from build123d import *

# Parameters (mm, degrees)
BOSS_EXTRUDE1_DEPTH  = 9.525
M8_CLEARANCE_HOLE1_D = 9
FILLET1_R            = 10
CHAMFER1_SIZE        = 1


with BuildPart() as part:
    # Sketch1 → Boss-Extrude1 (new body)
    with BuildSketch(Plane(origin=(0, 0, 0), x_dir=(1, 0, 0), z_dir=(0, 1, 0))):
        Polygon((-20, 90), (-20, -20), (60, -20), (60, 10), (20, 10), (20, 90), align=None)
    extrude(amount=BOSS_EXTRUDE1_DEPTH)

    # M8 Clearance Hole1 (through all)
    with Locations(Plane(origin=(0, 9.525, 0), x_dir=(1, 0, 0), z_dir=(0, 1, 0))):
        with Locations((0, 0), (40, 0)):
            Hole(M8_CLEARANCE_HOLE1_D / 2)

    # Fillet1
    fillet1_edges = [part.edges().sort_by_distance(p)[0] for p in [
        (20, 4.7625, -10),
    ]]
    fillet(fillet1_edges, radius=FILLET1_R)

    # Chamfer1
    chamfer1_edges = [part.edges().sort_by_distance(p)[0] for p in [
        (20, 4.7625, -90),
        (60, 4.7625, -10),
        (60, 4.7625, 20),
        (-20, 4.7625, 20),
        (-20, 4.7625, -90),
    ]]
    chamfer(chamfer1_edges, length=CHAMFER1_SIZE)


solid = part.part
Check sheet for the modelled part. Datum: model origin and axes. Units: mm. A direction names the side the tool comes from. Coordinates: 2 decimals unless noted, no trailing zeros. Loops run counter-clockwise (first coordinate to the right, second up) from the corner with the lowest first, then second, coordinate; pieces in that order, holes last. Notation, with made-up numbers: (3, 13) -> (10, 13) arc R33 cw to (10, 41) -> close; hole circle Ø1 at (22, 26.5). An arc over 180 degrees is marked (long way). Write item = value, one per line. Start each with the question number.
1. Section check D-D on x = 0. Record the cut outline in (y, z) (3 decimals), then the cut area to 3 significant figures.
2. Material ranges on line 1 (X direction, y = 4.5, z = 1.5); line 2 (X direction, y = 3.25, z = 2); line 3 (Z direction, x = 0, y = 5), recorded low to high.
3. Section check C-C on y = 5.25. Record the cut outline in (x, z).
4. Depth check by flat-ended pin: P1, Ø1.5, axis at y = 6, z = -67, coming from the +X side; P2, Ø1, axis at x = 46.5, y = 6.5, coming from the -Z side; P3, Ø5, axis at x = 28.5, y = 7.5, coming from the -Z side. Enter the tip coordinate at first touch or a pass-through.
5. Tool access check on faces 4 (the flat face through (20, 5, -54)), 5 (the flat face through (0, 5, -90)). Record the directions out of +Z, -Z, +X, -X, +Y, -Y that give a thin tool (end or side, any length) a straight path to the whole face; none if there is none.
6. Section check A-A on z = 0. Record the cut outline in (x, y) (3 decimals), then the cut area to 3 significant figures.
7. Draft check along X on faces 1 (the cylindrical face through (35.708, 4.696, -1.352)), 2 (the flat face through (-20, 5, -36)), 3 (the cylindrical face through (22.85, 4.83, -13.01)). Enter one of: released by +X, released by -X, zero draft, split by the parting line, or undercut.
8. Section check B-B on x = 40. Record the cut outline in (y, z) (3 decimals).
Responses:
q1.outline = (0, -90) -> (9.525, -90) -> (9.525, -4.5) -> (0, -4.5) -> close; (0, 4.5) -> (9.525, 4.5) -> (9.525, 20) -> (0, 20) -> close
q1.area = 962 mm2
q2.line_1 = -20 to -4.24, 4.24 to 35.76, 44.24 to 60
q2.line_2 = -20 to -4.03, 4.03 to 35.97, 44.03 to 60
q2.line_3 = -90 to -4.5, 4.5 to 20
q3.outline = (-20, -89) -> (-19, -90) -> (19, -90) -> (20, -89) -> (20, -20) arc R10 cw to (30, -10) -> (59, -10) -> (60, -9) -> (60, 19) -> (59, 20) -> (-19, 20) -> (-20, 19) -> close; hole circle Ø9 at (0, 0); hole circle Ø9 at (40, 0)
q4.P1 = 20
q4.P2 = -10
q4.P3 = -10.83
q5.face_4 = -Z, +X, +Y, -Y
q5.face_5 = -Z, +X, -X, +Y, -Y
q6.outline = (-20, 0) -> (-4.5, 0) -> (-4.5, 9.525) -> (-20, 9.525) -> close; (4.5, 0) -> (35.5, 0) -> (35.5, 9.525) -> (4.5, 9.525) -> close; (44.5, 0) -> (60, 0) -> (60, 9.525) -> (44.5, 9.525) -> close
q6.area = 591 mm2
q7.face_1 = undercut
q7.face_2 = released by -X
q7.face_3 = released by +X
q8.outline = (0, -10) -> (9.525, -10) -> (9.525, -4.5) -> (0, -4.5) -> close; (0, 4.5) -> (9.525, 4.5) -> (9.525, 20) -> (0, 20) -> close
